Work out the finished part from the listing and answer in its coordinate system (mm). A direction names the side the tool comes from. Round coordinates to 2 decimals unless told otherwise and drop trailing zeros. Order: outer loops, then holes, each group sorted by start corner. A loop starts at its lowest first (then second) coordinate and runs counter-clockwise, first axis right, second up. Notation, with made-up numbers: (85, 83.25) -> (92, 83.25) arc R25 cw to (92, 95.25) -> close; hole circle Ø11 at (24.5, -19). An arc over 180 degrees is marked (long way). Use a Markdown table: item, result. Add a question column.
Item 1: A cutting plane is placed at B-B, the plane z = 0.9. Determine the outline of the cut face in (x, y), plus the area to 3 significant figures.
Item 2: A cutting plane is placed at D-D, the plane x = -18. Determine the outline of the cut face in (y, z), plus the area to 3 significant figures.
Item 3: A tool of negligible diameter and unlimited length cuts with its end or side. For faces 1 (the flat face through (0, -4.5, 1)), 2 (the flat face through (0, -5, 0)), from which of +Z, -Z, +X, -X, +Y, -Y can it reach the whole face along a straight path? Write none if from no direction.
Item 4: For a pull along X with two mould halves and no side action, classify faces 3 (the flat face through (0, 4.5, 1)), 4 (the cylindrical face through (-4.769, 21.477, 0.986)), 5 (the flat face through (0, -5, 2)) as +X half, -X half, draft (parallel to the pull), parting line (faces both ways), or undercut.
Item 5: A cutting plane is placed at C-C, the plane y = 0. Determine the outline of the cut face in (x, z), plus the area to 3 significant figures.
Item 6: Flat-ended cylindrical pins translate along their axes: P1, Ø0.6, axis at x = 3, z = 1.5, coming from the +Y side; P2, Ø0.6, axis at y = 2, z = 0.5, coming from the +X side. Find the tip coordinate at first contact, or state that the pin passes through.
Item 7: Find the intervals of material crossed by L1, parallel to X at y = 0.5, z = 0.8; L2, parallel to Y at x = 0.5, z = 1.1; L3, parallel to X at y = -3, z = 1.45, in increasing order. Write a range as [from, to].
Item 8: A cutting plane is placed at A-A, the plane x = 0. Determine the outline of the cut face in (y, z).
Autodesk Inventor part; units mm, degrees
ref_plane "YZ Plane" through (0, 0, 0) normal (1, 0, 0) x (0, 1, 0)
ref_plane "XZ Plane" through (0, 0, 0) normal (0, 1, 0) x (-1, 0, 0)
ref_plane "XY Plane" through (0, 0, 0) normal (0, 0, 1) x (1, 0, 0)
ref_plane "Arbeitsebene1" through (0, 0, 0) normal (0, 0, 1) x (1, 0, 0)
sketch "Skizze1" plane through (0, 0, 0) normal (0, 0, 1) x (1, 0, 0)
  circle A0 centre (0, 0) radius 22
  point P0 (0, 0)
extrude "Extrusion1" add sketch "Skizze1" along normal blind 2
sketch "Skizze2" plane through (0, 0, 2) normal (0, 0, 1) x (1, 0, 0)
  circle A0 centre (-18, 0) radius 1.6
  circle A1 centre (18, 0) radius 1.6
  point P0 (0, 0)
  point P1 (19.0059, -0.5696)
hole "Bohrung1" at (-18, 0, 2) at (19.0059, -0.5696, 2) direction (0, 0, -1) diameter 3.2 end through all
sketch "Skizze3" plane through (0, 0, 2) normal (0, 0, 1) x (1, 0, 0)
  line L0 (6.5, -4.5) -> (-6.5, -4.5)
  line L1 (-6.5, -4.5) -> (-6.5, 4.5)
  line L2 (-6.5, 4.5) -> (6.5, 4.5)
  line L3 (6.5, 4.5) -> (6.5, -4.5)
  line L4 (6.5, -4.5) -> (-6.5, 4.5) construction
  line L5 (-6.5, -4.5) -> (6.5, 4.5) construction
  point P0 (0, 0)
  dimension "d9" = 13
  dimension "d10" = 9
extrude "Extrusion2" cut sketch "Skizze3" against normal blind 10
properties part number "led_deckel"
Reported:
| question | item | result |
|---|---|---|
| 1 | outline | circle Ø44 at (0, 0); hole circle Ø3.2 at (-18, 0); hole (-6.5, -4.5) -> (6.5, -4.5) -> (6.5, 4.5) -> (-6.5, 4.5) -> close; hole circle Ø3.2 at (19.01, -0.57) |
| 1 | area | 1,390 mm² |
| 2 | outline | (-12.65, 0) -> (-1.6, 0) -> (-1.6, 2) -> (-12.65, 2) -> close; (1.6, 0) -> (12.65, 0) -> (12.65, 2) -> (1.6, 2) -> close |
| 2 | area | 44.2 mm² |
| 3 | face 1 | +Z, -Z |
| 3 | face 2 | -Z, +X, -X, +Y, -Y |
| 4 | face 3 | undercut |
| 4 | face 4 | parting line |
| 4 | face 5 | draft |
| 5 | outline | (-22, 0) -> (-19.6, 0) -> (-19.6, 2) -> (-22, 2) -> close; (-16.4, 0) -> (-6.5, 0) -> (-6.5, 2) -> (-16.4, 2) -> close; (6.5, 0) -> (17.51, 0) -> (17.51, 2) -> (6.5, 2) -> close; (20.5, 0) -> (22, 0) -> (22, 2) -> (20.5, 2) -> close |
| 5 | area | 49.6 mm² |
| 6 | P1 | y = 21.83 |
| 6 | P2 | x = 21.93 |
| 7 | L1 | [-21.99, -19.52], [-16.48, -6.5], [6.5, 17.82], [20.2, 21.99] |
| 7 | L2 | [-21.99, -4.5], [4.5, 21.99] |
| 7 | L3 | [-21.79, -6.5], [6.5, 21.79] |
| 8 | outline | (-22, 0) -> (-4.5, 0) -> (-4.5, 2) -> (-22, 2) -> close; (4.5, 0) -> (22, 0) -> (22, 2) -> (4.5, 2) -> close |
